Read the model definition and answer for the solid it produces. Units are mm, in the model's axes. A direction names the side the tool comes from. Give positions to 0.01 mm unless a question says otherwise; leave off trailing zeros. Loops run counter-clockwise (first coordinate to the right, second up) from the corner with the lowest first, then second, coordinate; pieces in that order, holes last.
(1) Find section A-A, the plane x = 4.42. Write down the section's boundary in (y, z), then the cut area to 3 significant figures.
(2) Which of the six approach directions +Z, -Z, +X, -X, +Y, -Y give full straight-line access (tool end or side, diameter ignored) to faces 1 (the face through (10, 2, 2.569)), 2 (the face through (2, 2, 21.107)), 3 (the face through (17, 2, 21.107)), 4 (the face through (0.29, 2, 12))?
(3) Find section B-B, the plane z = 1.3. State how many separate pieces and enclosed holes the cut face has, then the cut area to 3 significant figures.
(4) Determine the mould class of faces 5 (the face through (9.669, 3.199, 23.155)), 6 (the face through (15.345, 2, 22)), 7 (the face through (16.632, 0.74, 1.192)) for opening direction X: pulls with the +X half, pulls with the -X half, needs draft (parallel to the pull), parting line crosses it, or undercut.
(5) Find section D-D, the plane y = 1.75. Write down the section's boundary in (x, z), then the cut area to 3 significant figures.
(6) Straight lines are drawn through the part: probe 1 along Y at (x, z) = (15.25, 2.25); probe 2 along Z at (x, y) = (2.5, 3); probe 3 along X at (y, z) = (3.35, 9.5). For each, find the intervals that lie inside material, in ascending order.
(7) Find section C-C, the plane x = 16.25. Write down the section's boundary in (y, z).
(8) Each of these flat-tipped pins is pushed along its axis until it touches: P1, Ø1.6, axis at y = 2.5, z = 15, coming from the -X side; P2, Ø0.6, axis at y = 2, z = 21.5, coming from the -X side; P3, Ø0.6, axis at y = 2.5, z = 22.5, coming from the +X side. Where does it stop, or does it pass through?
```python
from build123d import *

# Parameters (mm, degrees)
SKETCH1_W           = 19
SKETCH1_H           = 23.44
SKETCH1_R           = 0.5
BOSS_EXTRUDE1_DEPTH = 1.5
BOSS_EXTRUDE2_DEPTH = 2
FILLET1_R           = 1


with BuildPart() as part:
    # Sketch1 → Boss-Extrude1 (new body)
    with BuildSketch(Plane(origin=(0, 0, 0), x_dir=(1, 0, 0), z_dir=(0, 1, 0))):
        with Locations((9.5, -11.72)):
            Rectangle(SKETCH1_W, SKETCH1_H)
        with Locations(Location((1.88, -1.3, 0), (0, 0, 270))):
            Circle(SKETCH1_R, mode=Mode.SUBTRACT)
        with Locations(Location((4.42, -1.3, 0), (0, 0, 270))):
            Circle(SKETCH1_R, mode=Mode.SUBTRACT)
        with Locations(Location((6.96, -1.3, 0), (0, 0, 270))):
            Circle(SKETCH1_R, mode=Mode.SUBTRACT)
        with Locations(Location((9.5, -1.3, 0), (0, 0, 270))):
            Circle(SKETCH1_R, mode=Mode.SUBTRACT)
        with Locations(Location((12.04, -1.3, 0), (0, 0, 270))):
            Circle(SKETCH1_R, mode=Mode.SUBTRACT)
        with Locations(Location((14.58, -1.3, 0), (0, 0, 270))):
            Circle(SKETCH1_R, mode=Mode.SUBTRACT)
        with Locations(Location((17.12, -1.3, 0), (0, 0, 270))):
            Circle(SKETCH1_R, mode=Mode.SUBTRACT)
    extrude(amount=BOSS_EXTRUDE1_DEPTH)

    # Sketch3 → Boss-Extrude2 (add)
    with BuildSketch(Plane(origin=(0, 1.5, 0), x_dir=(1, 0, 0), z_dir=(0, 1, 0))):
        Polygon((3.832385917, -21.106985825), (3.832385917, -23.44), (15.344727023, -23.44), (15.344727023, -21.106985825), (18.591797592, -21.106985825), (18.591797592, -2.569164761), (0.290127115, -2.569164761), (0.290127115, -21.106985825), align=None)
    extrude(amount=BOSS_EXTRUDE2_DEPTH)

    # Fillet1
    fillet1_edges = [part.edges().sort_by_distance(p)[0] for p in [
        (9.58855647, 3.5, 23.44),
    ]]
    fillet(fillet1_edges, radius=FILLET1_R)


solid = part.part
```
Entries:
1. outline: (0, 0) - (1.5, 0) - (1.5, 0.8) - (0, 0.8) - close; (0, 1.8) - (1.5, 1.8) - (1.5, 2.57) - (3.5, 2.57) - (3.5, 22.44) arc R1 ccw to (2.5, 23.44) - (0, 23.44) - close
1. area: 75.2 mm2
2. face 1: -Z, +X, -X, +Y
2. face 2: +Z, -X, +Y
2. face 3: +Z, +X, +Y
2. face 4: +Z, -Z, -X, +Y
3. separate pieces: 8
3. enclosed holes: 0
3. area: 18.0 mm2
4. face 5: needs draft
4. face 6: pulls with the +X half
4. face 7: undercut
5. outline: (0.29, 2.57) - (18.59, 2.57) - (18.59, 21.11) - (15.34, 21.11) - (15.34, 23.44) - (3.83, 23.44) - (3.83, 21.11) - (0.29, 21.11) - close
5. area: 366 mm2
6. probe 1: y = 0 to 1.5
6. probe 2: z = 2.57 to 21.11
6. probe 3: x = 0.29 to 18.59
7. outline: (0, 0) - (1.5, 0) - (1.5, 2.57) - (3.5, 2.57) - (3.5, 21.11) - (1.5, 21.11) - (1.5, 23.44) - (0, 23.44) - close
8. P1: stops at x = 0.29
8. P2: stops at x = 3.83
8. P3: stops at x = 15.34
